The listing builds one solid part. Answer for the finished solid, in the listing's coordinates (mm). Face numbers are marked on the shaded views. A direction names the side the tool comes from. Coordinates: 2 decimals unless noted, no trailing zeros. Loops run counter-clockwise (first coordinate to the right, second up) from the corner with the lowest first, then second, coordinate; pieces in that order, holes last. Notation, with made-up numbers: (73, 27.25) -> (78, 27.25) arc R15 cw to (78, 53.25) -> close; hole circle Ø11 at (74, 82.25). An arc over 180 degrees is marked (long way). Answer in a Markdown table with one row per item.
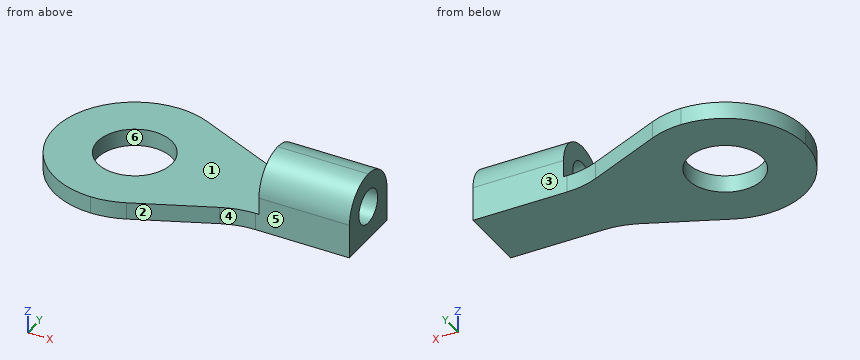
```python
from build123d import *

# Parameters (mm, degrees)
F0_R     = 1.85
F1_DEPTH = 0.85
F2_W     = 4.5
F2_H     = 3.4
F3_DEPTH = 2.55
F4_R     = 1.69999
F5_R     = 0.85
F6_DEPTH = 25


# Not quite as in the source:
# - a fillet or chamfer is up to 0.001 mm smaller than in the source, because OpenCascade refuses the exact size


with BuildPart() as f1:
    # F0 (on Top) → F1 (new body)
    with BuildSketch(Plane.XY):
        with BuildLine():
            Line((10.9356666081, 2.3), (15.6, 2.3))
            Line((15.6, 2.3), (15.6, 5.7))
            Line((15.6, 5.7), (10.9356666081, 5.7))
            ThreePointArc((10.9356666081, 5.7), (10.117660762, 5.7845349656), (9.3342299639, 6.0345667821))
            Line((9.3342299639, 6.0345667821), (5.6014366442, 7.6654332179))
            ThreePointArc((5.6014366442, 7.6654332179), (4.8180058461, 7.9154650344), (4, 8))
            ThreePointArc((4, 8), (1.1715728753, 6.8284271247), (0, 4))
            ThreePointArc((0, 4), (1.1715728753, 1.1715728753), (4, 0))
            ThreePointArc((4, 0), (4.8180058461, 0.0845349656), (5.6014366442, 0.3345667821))
            Line((5.6014366442, 0.3345667821), (9.3342299639, 1.9654332179))
            ThreePointArc((9.3342299639, 1.9654332179), (10.117660762, 2.2154650344), (10.9356666081, 2.3))
        make_face()
        with Locations((4, 4)):
            Circle(F0_R, mode=Mode.SUBTRACT)
    extrude(amount=F1_DEPTH)

    # F2 (on face) → F3 (join)
    with BuildSketch(Plane.XY.offset(0.85)):
        with Locations((13.35, 4)):
            Rectangle(F2_W, F2_H)
    extrude(amount=F3_DEPTH)

    # F4 (radius 1.7 in the source; OpenCascade refuses exactly that, so slightly less here)
    f4_edges = [f1.edges().sort_by_distance(p)[0] for p in [
        (13.35, 5.7, 3.4),
        (13.35, 2.3, 3.4),
    ]]
    fillet(f4_edges, radius=F4_R)

    # F5 (on face) → F6 (cut)
    with BuildSketch(Plane.YZ.offset(15.6)):
        with Locations((4, 1.7)):
            Circle(F5_R)
    extrude(amount=-F6_DEPTH, mode=Mode.SUBTRACT)


solid = f1.part
```
Item 1: Find the intervals of material crossed by probe 1 along Y at (x, z) = (4, 0.5); probe 2 along X at (y, z) = (4, 0.45); probe 3 along Z at (x, y) = (13, 4), in increasing order.
Findings below:
| item | result |
|---|---|
| probe 1 | y = 0 to 2.15, 5.85 to 8 |
| probe 2 | x = 0 to 2.15, 5.85 to 15.6 |
| probe 3 | z = 0 to 0.85, 2.55 to 3.4 |
Item 2: A cutting plane is placed at C-C, the plane y = 5.25. Determine the outline of the cut face in (x, z).
Findings below:
| item | result |
|---|---|
| outline | (0.2, 0) -> (2.64, 0) -> (2.64, 0.85) -> (0.2, 0.85) -> close; (5.36, 0) -> (15.6, 0) -> (15.6, 2.85) -> (11.1, 2.85) -> (11.1, 0.85) -> (5.36, 0.85) -> close |
Item 3: A tool of negligible diameter and unlimited length cuts with its end or side. For the marked faces 1, 2 and 3, from which of +Z, -Z, +X, -X, +Y, -Y can it reach the whole face along a straight path? Write none if from no direction.
Findings below:
| item | result |
|---|---|
| face 1 | +Z, -X, +Y, -Y |
| face 2 | +Z, -Z, +X, -Y |
| face 3 | +Z, -Z, +X, +Y |
Item 4: A cutting plane is placed at B-B, the plane z = 0.4. Determine the outline of the cut face in (x, y), plus the area to 3 significant figures.
Findings below:
| item | result |
|---|---|
| outline | (5.6, 0.33) -> (9.33, 1.97) arc R4 cw to (10.94, 2.3) -> (15.6, 2.3) -> (15.6, 5.7) -> (10.94, 5.7) arc R4 cw to (9.33, 6.03) -> (5.6, 7.67) arc R4 ccw (long way) to start; hole circle Ø3.7 at (4, 4) |
| area | 69.8 mm2 |
Item 5: Determine the mould class of the marked faces 4, 5 and 6 for opening direction X: +X half, -X half, draft (parallel to the pull), parting line (faces both ways), or undercut.
Findings below:
| item | result |
|---|---|
| face 4 | +X half |
| face 5 | draft |
| face 6 | undercut |
Item 6: Flat-ended cylindrical pins translate along their axes: pin 1 Ø0.5 at (x, z) = (13.5, 0.5) entering from -Y; pin 2 Ø0.9 at (x, z) = (13, 1) entering from +Y; pin 3 Ø0.8 at (y, z) = (5, 2.5) entering from -X. Find the tip coordinate at first contact, or state that the pin passes through.
Findings below:
| item | result |
|---|---|
| pin 1 | stops at y = 2.3 |
| pin 2 | stops at y = 5.7 |
| pin 3 | stops at x = 11.1 |
Item 7: A cutting plane is placed at D-D, the plane z = 1.55. Determine the outline of the cut face in (x, y).
Findings below:
| item | result |
|---|---|
| outline | (11.1, 2.3) -> (15.6, 2.3) -> (15.6, 3.16) -> (11.1, 3.16) -> close; (11.1, 4.84) -> (15.6, 4.84) -> (15.6, 5.7) -> (11.1, 5.7) -> close |
